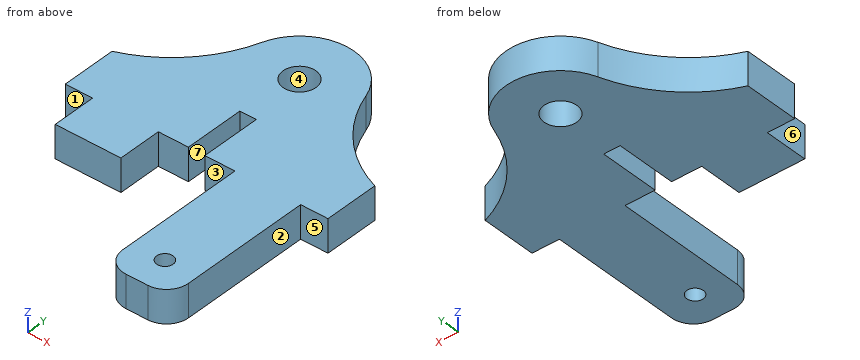
from build123d import *

# Parameters (mm, degrees)
SKETCH1_R           = 1.5
SKETCH1_R_2         = 0.75
BOSS_EXTRUDE1_DEPTH = 3
SKETCH2_W           = 2.5
SKETCH2_H           = 4
CUT_EXTRUDE1_DEPTH  = 10
SKETCH3_W           = 3.5
SKETCH3_H           = 4
BOSS_EXTRUDE2_DEPTH = 3
SKETCH4_W           = 2.5
SKETCH4_H           = 14
CUT_EXTRUDE2_DEPTH  = 10
FILLET1_R           = 2


with BuildPart() as part:
    # Sketch1 → Boss-Extrude1 (new body)
    with BuildSketch(Plane.XY):
        with BuildLine():
            Line((-0.75, -11), (-7, -11))
            Line((-7, -11), (-7, -15))
            Line((-7, -15), (-12, -15))
            Line((-12, -15), (-12, -11))
            Line((-12, -11), (-12, -6))
            ThreePointArc((-12, -6), (-7.512319363, -3.05842228), (-4.755323166, 1.544960058))
            ThreePointArc((-4.755323166, 1.544960058), (0, 5), (4.755323166, 1.544960058))
            ThreePointArc((4.755323166, 1.544960058), (7.512319363, -3.05842228), (12, -6))
            Line((12, -6), (12, -25))
            Line((12, -25), (3.5, -25))
            Line((3.5, -25), (3.5, -11))
            Line((3.5, -11), (0.75, -11))
            Line((0.75, -11), (0.75, -5.5))
            Line((0.75, -5.5), (-0.75, -5.5))
            Line((-0.75, -5.5), (-0.75, -11))
        make_face()
        Circle(SKETCH1_R, mode=Mode.SUBTRACT)
        with Locations((6.5, -22)):
            Circle(SKETCH1_R_2, mode=Mode.SUBTRACT)
    extrude(amount=BOSS_EXTRUDE1_DEPTH)

    # Sketch2 → Cut-Extrude1 (cut)
    with BuildSketch(Plane.XY.offset(3)):
        with Locations((-10.75, -13)):
            Rectangle(SKETCH2_W, SKETCH2_H)
    extrude(amount=-CUT_EXTRUDE1_DEPTH, mode=Mode.SUBTRACT)

    # Sketch3 → Boss-Extrude2 (add)
    with BuildSketch(Plane.XY.offset(3)):
        with Locations((-5.25, -13)):
            Rectangle(SKETCH3_W, SKETCH3_H)
    extrude(amount=-BOSS_EXTRUDE2_DEPTH)

    # Sketch4 → Cut-Extrude2 (cut)
    with BuildSketch(Plane.XY.offset(3)):
        with Locations((10.75, -18)):
            Rectangle(SKETCH4_W, SKETCH4_H)
    extrude(amount=-CUT_EXTRUDE2_DEPTH, mode=Mode.SUBTRACT)

    # Fillet1
    fillet1_edges = [part.edges().sort_by_distance(p)[0] for p in [
        (3.5, -25, 1.5),
        (9.5, -25, 1.5),
    ]]
    fillet(fillet1_edges, radius=FILLET1_R)


solid = part.part
For this review, take the finished solid that the model builds, in its own axes (mm). Face numbers are marked on the shaded views. A direction names the side the tool comes from. Round coordinates to 2 decimals unless told otherwise and drop trailing zeros. Write each loop counter-clockwise with the first axis right and the second up, starting at its lowest first coordinate (ties: lowest second). Pieces come first, ordered by that corner, then holes. Notation, with made-up numbers: (35.25, 40.25) - (43.25, 40.25) arc R34 ccw to (43.25, 77.25) - close; hole circle Ø11 at (71.25, -24). An arc over 180 degrees is marked (long way). Use a Markdown table: item, result.
Q1. We need section A-A (y = -8.75). Give the boundary of the cut face in (x, z).
Derived:
| item | result |
|---|---|
| outline | (-12, 0) - (-0.75, 0) - (-0.75, 3) - (-12, 3) - close; (0.75, 0) - (12, 0) - (12, 3) - (0.75, 3) - close |
Q2. Machinability: for the marked faces 1, 2, 3 and 4, which of the approach directions +Z, -Z, +X, -X, +Y, -Y give a long, thin tool a straight path to every point of the face, cutting with its end or side? Answer none if there is none.
Derived:
| item | result |
|---|---|
| face 1 | +Z, -Z, -X, -Y |
| face 2 | +Z, -Z, +X, -Y |
| face 3 | +Z, -Z, -Y |
| face 4 | +Z, -Z |
Q3. We need section C-C (x = 0). Give the boundary of the cut face in (y, z).
Derived:
| item | result |
|---|---|
| outline | (-5.5, 0) - (-1.5, 0) - (-1.5, 3) - (-5.5, 3) - close; (1.5, 0) - (5, 0) - (5, 3) - (1.5, 3) - close |
Q4. Clearance check with flat-ended pins moving along their axes: pin 1 (0.9 mm diameter, centred on y = -12.5, z = 1.5, fed in from -X); pin 2 (1 mm diameter, centred on y = 1, z = 2, fed in from -X); pin 3 (0.8 mm diameter, centred on x = 3, z = 1, fed in from -Y). State where each tip first meets the part, or that it passes through.
Derived:
| item | result |
|---|---|
| pin 1 | stops at x = -9.5 |
| pin 2 | stops at x = -5.15 |
| pin 3 | stops at y = -11 |
Q5. We need section D-D (y = -19.5). Give the boundary of the cut face in (x, z).
Derived:
| item | result |
|---|---|
| outline | (3.5, 0) - (9.5, 0) - (9.5, 3) - (3.5, 3) - close |
Q6. Wall thickness on line 1 along Y through (x, z) = (6.5, 1.3); line 2 along X through (y, z) = (-0.5, 0.8); line 3 along X through (y, z) = (-20, 1.45): over which ranges is each line inside the solid? List them lowest first.
Derived:
| item | result |
|---|---|
| line 1 | y = -25 to -22.75, -21.25 to -1.86 |
| line 2 | x = -5.64 to -1.41, 1.41 to 5.64 |
| line 3 | x = 3.5 to 9.5 |
Q7. We need section B-B (z = 0.4). Give the boundary of the cut face in (x, y), plus the area to 3 significant figures.
Derived:
| item | result |
|---|---|
| outline | (-12, -11) - (-9.5, -11) - (-9.5, -15) - (-3.5, -15) - (-3.5, -11) - (-0.75, -11) - (-0.75, -5.5) - (0.75, -5.5) - (0.75, -11) - (3.5, -11) - (3.5, -23) arc R2 ccw to (5.5, -25) - (7.5, -25) arc R2 ccw to (9.5, -23) - (9.5, -11) - (12, -11) - (12, -6) arc R12 cw to (4.76, 1.54) arc R5 ccw to (-4.76, 1.54) arc R12 cw to (-12, -6) - close; hole circle Ø3 at (0, 0); hole circle Ø1.5 at (6.5, -22) |
| area | 343 mm2 |
Q8. The part is to be moulded in two halves that separate along X. For the marked faces 5, 6 and 7, say which applies: pulls with the +X half, pulls with the -X half, needs draft (parallel to the pull), parting line crosses it, or undercut.
Derived:
| item | result |
|---|---|
| face 5 | needs draft |
| face 6 | pulls with the -X half |
| face 7 | undercut |
